from build123d import *

# Parameters (mm, degrees)
SKETCH1_R               = 2.45
BOSS_EXTRUDE1_DEPTH     = 10
SKETCH2_R               = 5.95
BOSS_EXTRUDE2_DEPTH     = 35
SKETCH4_W               = 11.9
SKETCH4_H               = 15
CUT_EXTRUDE1_DEPTH      = 2.5
CUT_EXTRUDE2_DEPTH      = 46.779962866
CUT_EXTRUDE2_DEPTH_BACK = 46.779962866
SKETCH5_R               = 1.6
FILLET1_R               = 4
FILLET2_R               = 3
SKETCH6_R               = 1.15
CUT_EXTRUDE3_DEPTH      = 15


with BuildPart() as part:
    # Sketch1 → Boss-Extrude1 (new body)
    with BuildSketch(Plane(origin=(0, 0, 0), x_dir=(1, 0, 0), z_dir=(0, 1, 0))):
        with Locations(Location((0, 0, 0), (0, 0, 270))):
            Circle(SKETCH1_R)
    extrude(amount=BOSS_EXTRUDE1_DEPTH)

    # Sketch2 → Boss-Extrude2 (add)
    with BuildSketch(Plane(origin=(0, 10, 0), x_dir=(1, 0, 0), z_dir=(0, 1, 0))):
        with Locations(Location((0, 0, 0), (0, 0, 270))):
            Circle(SKETCH2_R)
    extrude(amount=BOSS_EXTRUDE2_DEPTH)

    # Sketch4 → Cut-Extrude1 (cut, symmetric)
    with BuildSketch(Plane(origin=(0, 0, 0), x_dir=(0, 0, -1), z_dir=(1, 0, 0))):
        with Locations((0, 37.5)):
            Rectangle(SKETCH4_W, SKETCH4_H)
    extrude(amount=CUT_EXTRUDE1_DEPTH, both=True, mode=Mode.SUBTRACT)

    # Sketch5 → Cut-Extrude2 (cut, two sides: drawn at the far end of the back side and taken through both)
    with BuildSketch(Plane(origin=(0, 0, 0), x_dir=(0, 0, -1), z_dir=(1, 0, 0)).offset(-CUT_EXTRUDE2_DEPTH_BACK)):
        with Locations((0, 38)):
            Circle(SKETCH5_R)
    extrude(amount=CUT_EXTRUDE2_DEPTH + CUT_EXTRUDE2_DEPTH_BACK, mode=Mode.SUBTRACT)

    # Fillet1
    # the kernel refuses this fillet: 4 mm, written as the material it takes off along each edge
    with BuildSketch(Plane(origin=(0, 45, 0), x_dir=(-0.9484971142590468, 0, 0.31678577026479715), z_dir=(-0.31678577026479715, 0, -0.9484971142590468))) as fillet1_piece_1:
        with BuildLine():
            CenterArc((5.95 - FILLET1_R, -FILLET1_R), FILLET1_R, 0, 90)
            Line((5.95 - FILLET1_R, 0), (5.95, 0))
            Line((5.95, 0), (5.95, -FILLET1_R))
        make_face()
    revolve(axis=Axis((0, 45, 0), (0, 1, 0)), revolution_arc=323.062694348, mode=Mode.SUBTRACT)
    with BuildSketch(Plane(origin=(0, 45, 0), x_dir=(0.948497114259044, 0, -0.31678577026480526), z_dir=(0.31678577026480526, 0, 0.948497114259044))) as fillet1_piece_2:
        with BuildLine():
            CenterArc((5.95 - FILLET1_R, -FILLET1_R), FILLET1_R, 0, 90)
            Line((5.95 - FILLET1_R, 0), (5.95, 0))
            Line((5.95, 0), (5.95, -FILLET1_R))
        make_face()
    revolve(axis=Axis((0, 45, 0), (0, 1, 0)), revolution_arc=323.062694348, mode=Mode.SUBTRACT)

    # Fillet2
    fillet2_edges = [part.edges().sort_by_distance(p)[0] for p in [
        (0, 30, -5.95),
        (1.279967228, 30, 5.810695646),
    ]]
    fillet(fillet2_edges, radius=FILLET2_R)

    # Sketch6 → Cut-Extrude3 (cut)
    with BuildSketch(Plane(origin=(-0.011753066, 0, 5.949988392), x_dir=(0.9999980490826653, 0, 0.0019753052582657496), z_dir=(-0.0019753052582657496, 0, 0.9999980490826653))):
        with Locations((-0.258432266, 24)):
            Circle(SKETCH6_R)
    extrude(amount=-CUT_EXTRUDE3_DEPTH, mode=Mode.SUBTRACT)


solid = part.part
Geometry check sheet. Reference: the model listing, model coordinates, mm. A direction names the side the tool comes from. Give positions to 0.01 mm unless a question says otherwise; leave off trailing zeros. Loops run counter-clockwise (first coordinate to the right, second up) from the corner with the lowest first, then second, coordinate; pieces in that order, holes last. Notation, with made-up numbers: M 17.25,5 L 53.25,5 A4 cw 53.25,9 Z; hole C 20.5,-12 d2. An arc over 180 degrees is marked long. Answer as a JSON object with one key per item and string values. Group by question number.
Item 1: Sectioned sample at C-C on z = 0. Give the number of separate pieces and of enclosed holes in the cut face, plus the area to 3 significant figures.
Item 2: Sectioned sample at B-B on y = 38. Record the boundary of the cut face in (x, z).
Item 3: Gauge pin test, flat ends, axial feed: pin 1 (3 mm diameter, centred on y = 23, z = -4.5, fed in from -X); pin 2 (6 mm diameter, centred on x = -3.5, y = 30, fed in from -Z); pin 3 (4 mm diameter, centred on x = 0, z = -0.5, fed in from +Y). Record the tip position at first contact, or that the pin passes through.
Item 4: Material ranges on L1, parallel to X at y = 40, z = 2.5; L2, parallel to X at y = 32, z = 0.25; L3, parallel to Y at x = -0.25, z = 3, recorded low to high.
Item 5: Sectioned sample at D-D on y = 8.5. Record the boundary of the cut face in (x, z), plus the area to 3 significant figures.
Item 6: Sectioned sample at A-A on y = 33.5. Record the boundary of the cut face in (x, z).
Item 7: Mould release check, pull along Y, two halves, no side actions. Record for faces 3 (the cylindrical face through (4.2, 37.39, -1.48)), 4 (the flat face through (-2.5, 36, 0)), 5 (the flat face through (0, 30, 0)), 6 (the flat face through (0, 10, 3)): pulls with the +Y half, pulls with the -Y half, needs draft (parallel to the pull), parting line crosses it, or undercut.
Item 8: Access from +Z, -Z, +X, -X, +Y, -Y to the whole of each face (thin tool, end or side, straight path). Record for faces 1 (the flat face through (0, 0, 0)), 2 (the cylindrical face through (0.736, 4.93, 2.337)).
Findings below:
{
 "1": {"separate pieces": "3", "enclosed holes": "1", "area": "357 mm2"},
 "2": {"outline": "M -5.73,-1.6 A5.95 ccw -2.5,-5.4 L -2.5,-1.6 Z; M -5.73,1.6 L -2.5,1.6 L -2.5,5.4 A5.95 ccw Z; M 2.5,-5.4 A5.95 ccw 5.73,-1.6 L 2.5,-1.6 Z; M 2.5,1.6 L 5.73,1.6 A5.95 ccw 2.5,5.4 Z"},
 "3": {"pin 1": "x = -5.14", "pin 2": "z = -5.66", "pin 3": "y = 30"},
 "4": {"L1": "-5.4 to -2.5, 2.5 to 5.4", "L2": "-5.94 to -2.5, 2.5 to 5.94", "L3": "10 to 22.85, 25.15 to 30"},
 "5": {"outline": "C 0,0 d4.9", "area": "18.9 mm2"},
 "6": {"outline": "M -2.5,-5.4 L -2.5,5.4 A5.95 ccw Z; M 2.5,-5.4 A5.95 ccw 2.5,5.4 Z"},
 "7": {"face 3": "undercut", "face 4": "needs draft", "face 5": "pulls with the +Y half", "face 6": "pulls with the -Y half"},
 "8": {"face 1": "+Z, -Z, +X, -X, -Y", "face 2": "-Y"}
}
